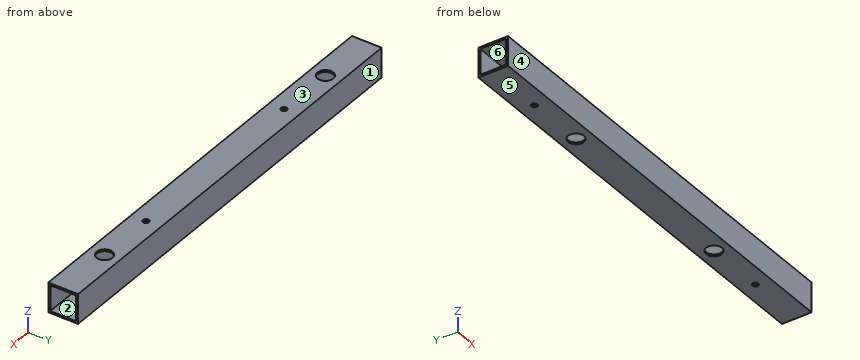
from build123d import *

# Parameters (mm, degrees)
SKETCH_1_W          = 15
SKETCH_1_H          = 15
SKETCH_1_W_2        = 13
SKETCH_1_H_2        = 13
EXTRUDE_1_DEPTH     = 220
SKETCH_2_R          = 1.5
CUT_EXTRUDE_4_DEPTH = 221.638278637
SKETCH_5_R          = 4
CUT_EXTRUDE_5_DEPTH = 10
SKETCH_6_R          = 4
CUT_EXTRUDE_6_DEPTH = 10


with BuildPart() as part:
    # 草图1 → 凸台-拉伸1 (new body)
    with BuildSketch(Plane(origin=(0, 0, 0), x_dir=(0, 0, -1), z_dir=(1, 0, 0))):
        Rectangle(SKETCH_1_W, SKETCH_1_H)
        Rectangle(SKETCH_1_W_2, SKETCH_1_H_2, mode=Mode.SUBTRACT)
    extrude(amount=EXTRUDE_1_DEPTH)

    # 草图2 → 切除-拉伸4 (cut, through all)
    with BuildSketch(Plane(origin=(0, 0, -7.5), x_dir=(-1, 0, 0), z_dir=(0, 0, -1))):
        with Locations((-30, 0)):
            Circle(SKETCH_2_R)
        with Locations((-60, 0)):
            Circle(SKETCH_2_R)
        with Locations(Location((-160, 0, 0), (0, 0, 270))):
            Circle(SKETCH_2_R)
        with Locations(Location((-190, 0, 0), (0, 0, 270))):
            Circle(SKETCH_2_R)
    extrude(amount=-CUT_EXTRUDE_4_DEPTH, mode=Mode.SUBTRACT)

    # 草图5 → 切除-拉伸5 (cut)
    with BuildSketch(Plane(origin=(0, 0, -7.5), x_dir=(-1, 0, 0), z_dir=(0, 0, -1))):
        with Locations((-160, 0)):
            Circle(SKETCH_5_R)
        with Locations((-60, 0)):
            Circle(SKETCH_5_R)
    extrude(amount=-CUT_EXTRUDE_5_DEPTH, mode=Mode.SUBTRACT)

    # 草图6 → 切除-拉伸6 (cut)
    with BuildSketch(Plane.XY.offset(7.5)):
        with Locations((190, 0)):
            Circle(SKETCH_6_R)
        with Locations((30, 0)):
            Circle(SKETCH_6_R)
    extrude(amount=-CUT_EXTRUDE_6_DEPTH, mode=Mode.SUBTRACT)


solid = part.part
Here's how the part is built. I have some questions about the finished solid (model axes, mm). Face numbers are marked on the shaded views. A direction names the side the tool comes from. Coordinates: 2 decimals unless noted, no trailing zeros. Order: outer loops, then holes, each group sorted by start corner. A loop starts at its lowest first (then second) coordinate and runs counter-clockwise, first axis right, second up. Notation, with made-up numbers: M -33,6 L 0,6 A20 cw 0,37 Z; hole C -4,54 d8. An arc over 180 degrees is marked long. Answer as CSV lines item,"result". Start each with the question number.
1. I want a section at B-B, the plane x = 23.5. Write out the boundary of the cut face in (y, z).
2. We'd pull the mould along Y, two halves only. Please class the marked faces 1, 2, 3 and 4: released by +Y, released by -Y, zero draft, split by the parting line, or undercut.
3. For pin 1 (2 mm diameter, centred on y = -6, z = -4.5, fed in from +X); pin 2 (6.5 mm diameter, centred on x = 160, y = 0, fed in from -Z); pin 3 (4 mm diameter, centred on x = 190, y = 0, fed in from +Z), each with a flat end and sliding along its axis, tell me the tip position at first contact or that it passes through.
4. On a 3-axis mill with a long thin cutter (end or side, diameter ignored), from which of +Z, -Z, +X, -X, +Y, -Y can I reach the whole of each face in a straight line? I mean the marked faces 5 and 6. Say none if no direction works.
5. I want a section at A-A, the plane z = -3.5. Write out the boundary of the cut face in (x, y).
6. I need wall thicknesses on line 1 (Y direction, x = 211, z = 0.25); line 2 (Y direction, x = 60, z = 7.15). Which ranges of each line are inside material? Lowest first, please. Write a range as [from, to].
Recorded:
1,outline,"M -7.5,-7.5 L 7.5,-7.5 L 7.5,7.5 L -7.5,7.5 Z; hole M -6.5,-6.5 L 6.5,-6.5 L 6.5,6.5 L -6.5,6.5 Z"
2,face 1,"released by +Y"
2,face 2,"undercut"
2,face 3,"zero draft"
2,face 4,"released by -Y"
3,pin 1,"stops at x = 220"
3,pin 2,"stops at z = 6.5"
3,pin 3,"stops at z = -6.5"
4,face 5,"-Z, +X, -X, +Y, -Y"
4,face 6,"+X, -X"
5,outline,"M 0,-7.5 L 220,-7.5 L 220,-6.5 L 0,-6.5 Z; M 0,6.5 L 220,6.5 L 220,7.5 L 0,7.5 Z"
6,line 1,"y = [-7.5, -6.5], [6.5, 7.5]"
6,line 2,"y = [-7.5, -1.5], [1.5, 7.5]"
